```python
from build123d import *

# Parameters (mm, degrees)
SKETCH2_R           = 12.7
BOSS_EXTRUDE1_DEPTH = 38.1
SKETCH3_R           = 19.05
BOSS_EXTRUDE2_DEPTH = 12.7
HOLE1_D             = 16.002
CHAMFER1_SIZE       = 1.524


with BuildPart() as part:
    # Sketch2 → Boss-Extrude1 (new, symmetric)
    with BuildSketch(Plane(origin=(0, 0, 0), x_dir=(1, 0, 0), z_dir=(0, 1, 0))):
        with Locations(Location((0, 0, 0), (0, 0, 90))):
            Circle(SKETCH2_R)
    extrude(amount=BOSS_EXTRUDE1_DEPTH, both=True)

    # Sketch3 → Boss-Extrude2 (add)
    with BuildSketch(Plane(origin=(0, 38.1, 0), x_dir=(1, 0, 0), z_dir=(0, 1, 0))):
        with Locations(Location((0, 0, 0), (0, 0, 270))):
            Circle(SKETCH3_R)
    extrude(amount=-BOSS_EXTRUDE2_DEPTH)

    # Hole1 (through all)
    with Locations(Plane(origin=(0, 38.1, 0), x_dir=(1, 0, 0), z_dir=(0, 1, 0))):
        with Locations((0, 0)):
            Hole(HOLE1_D / 2)

    # Chamfer1
    chamfer1_edges = [part.edges().sort_by_distance(p)[0] for p in [
        (0, -38.1, 12.7),
    ]]
    chamfer(chamfer1_edges, length=CHAMFER1_SIZE)


solid = part.part
```
Check sheet for the modelled part. Datum: model origin and axes. Units: mm. A direction names the side the tool comes from. Give positions to 0.01 mm unless a question says otherwise; leave off trailing zeros. Write each loop counter-clockwise with the first axis right and the second up, starting at its lowest first coordinate (ties: lowest second). Pieces come first, ordered by that corner, then holes. Notation, with made-up numbers: (-18, -21.75) - (38, -21.75) arc R25 ccw to (38, 13.25) - close; hole circle Ø10 at (8.5, 65). An arc over 180 degrees is marked (long way). Answer as a JSON object with one key per item and string values. Group by question number.
1) Sectioned sample at C-C (y = -7). Record the cut outline in (x, z), then the cut area to 3 significant figures.
2) Sectioned sample at D-D (x = 16.5). Record the cut outline in (y, z), then the cut area to 3 significant figures.
3) Depth check by flat-ended pin: P1, Ø12, axis at y = -25.5, z = -7.5, coming from the -X side; P2, Ø4, axis at x = -5.5, y = -2, coming from the -Z side; P3, Ø6, axis at y = -13.5, z = 8.5, coming from the -X side. Enter the tip coordinate at first touch or a pass-through.
4) Sectioned sample at A-A (z = 0). Record the cut outline in (x, y).
5) Thickness scan on probe 1 along X at (y, z) = (-34, -4.5); probe 2 along Z at (x, y) = (3, 12); probe 3 along Y at (x, z) = (3, -17). Record the ranges inside material, lowest first. Write a range as from..to.
6) Release check for a two-part mould opening along X. For faces 3 (the face through (1.73, -0.53, 7.81)), 4 (the face through (-8, -38.1, 3)), 5 (the face through (-11.59, 31.84, -15.12)) record: pulls with the +X half, pulls with the -X half, needs draft (parallel to the pull), parting line crosses it, or undercut.
7) Access from +Z, -Z, +X, -X, +Y, -Y to the whole of each face (thin tool, end or side, straight path). Record for faces 1 (the face through (7.7, -5.2, 10.1)), 2 (the face through (0.3, 38.1, 8.2)).
8) Sectioned sample at B-B (x = 0). Record the cut outline in (y, z).
Geometry results:
{
 "1": {"outline": "circle Ø25.4 at (0, 0); hole circle Ø16 at (0, 0)", "area": "306 mm^2"},
 "2": {"outline": "(25.4, -9.52) - (38.1, -9.52) - (38.1, 9.52) - (25.4, 9.52) - close", "area": "242 mm^2"},
 "3": {"P1": "stops at x = -12.61", "P2": "stops at z = -12.21", "P3": "stops at x = -11.45"},
 "4": {"outline": "(-19.05, 25.4) - (-12.7, 25.4) - (-12.7, -36.58) - (-11.18, -38.1) - (-8, -38.1) - (-8, 38.1) - (-19.05, 38.1) - close; (8, -38.1) - (11.18, -38.1) - (12.7, -36.58) - (12.7, 25.4) - (19.05, 25.4) - (19.05, 38.1) - (8, 38.1) - close"},
 "5": {"probe 1": "x = -11.88..-6.62, 6.62..11.88", "probe 2": "z = -12.34..-7.42, 7.42..12.34", "probe 3": "y = 25.4..38.1"},
 "6": {"face 3": "undercut", "face 4": "needs draft", "face 5": "parting line crosses it"},
 "7": {"face 1": "-Y", "face 2": "+Z, -Z, +X, -X, +Y"},
 "8": {"outline": "(-38.1, -11.18) - (-36.58, -12.7) - (25.4, -12.7) - (25.4, -19.05) - (38.1, -19.05) - (38.1, -8) - (-38.1, -8) - close; (-38.1, 8) - (38.1, 8) - (38.1, 19.05) - (25.4, 19.05) - (25.4, 12.7) - (-36.58, 12.7) - (-38.1, 11.18) - close"}
}
